```python
from build123d import *

# Parameters (mm, degrees)
BOSS_EXTRUDE1_DEPTH = 5
CUT_EXTRUDE1_DEPTH  = 2
SKETCH3_R           = 10
CUT_EXTRUDE4_DEPTH  = 73.034713854
BOSS_EXTRUDE2_START = 2
SKETCH5_R           = 15
SKETCH5_R_2         = 10
BOSS_EXTRUDE2_DEPTH = 2


with BuildPart() as part:
    # Sketch1 → Boss-Extrude1 (new, symmetric)
    with BuildSketch(Plane(origin=(0, 0, 0), x_dir=(1, 0, 0), z_dir=(0, 1, 0))):
        with BuildLine():
            Line((-28.618176043, 9), (-14.309088021, 54.5))
            ThreePointArc((-14.309088021, 54.5), (0, 65), (14.309088021, 54.5))
            Line((14.309088021, 54.5), (28.618176043, 9))
            ThreePointArc((28.618176043, 9), (0, -30), (-28.618176043, 9))
        make_face()
    extrude(amount=BOSS_EXTRUDE1_DEPTH, both=True)

    # Sketch2 → Cut-Extrude1 (cut)
    with BuildSketch(Plane(origin=(0, 5, 0), x_dir=(1, 0, 0), z_dir=(0, 1, 0))):
        with BuildLine():
            Line((-9.539392014, 53), (-23.848480035, 7.5))
            ThreePointArc((-23.848480035, 7.5), (0, -25), (23.848480035, 7.5))
            Line((23.848480035, 7.5), (9.539392014, 53))
            ThreePointArc((9.539392014, 53), (0, 60), (-9.539392014, 53))
        make_face()
    cut_extrude1 = extrude(amount=-CUT_EXTRUDE1_DEPTH, mode=Mode.SUBTRACT)

    # Mirror1: Cut-Extrude1 across plane
    add(cut_extrude1.mirror(Plane.ZX), mode=Mode.SUBTRACT)

    # Sketch3 → Cut-Extrude4 (cut, through all)
    with BuildSketch(Plane(origin=(0, 3, 0), x_dir=(1, 0, 0), z_dir=(0, 1, 0))):
        with Locations(Location((0, 0, 0), (0, 0, 270))):
            Circle(SKETCH3_R)
    extrude(amount=-CUT_EXTRUDE4_DEPTH, mode=Mode.SUBTRACT)

    # Sketch5 → Boss-Extrude2 (add)
    with BuildSketch(Plane(origin=(0, 3, 0), x_dir=(1, 0, 0), z_dir=(0, 1, 0)).offset(BOSS_EXTRUDE2_START)):
        with Locations(Location((0, 0, 0), (0, 0, 270))):
            Circle(SKETCH5_R)
        with Locations(Location((0, 0, 0), (0, 0, 270))):
            Circle(SKETCH5_R_2, mode=Mode.SUBTRACT)
    boss_extrude2 = extrude(amount=-BOSS_EXTRUDE2_DEPTH)

    # Mirror2: Boss-Extrude2 across plane
    add(boss_extrude2.mirror(Plane.ZX))


solid = part.part
```
Geometry: final body of the model. Coordinates: model frame, mm. A direction names the side the tool comes from. Coordinates: 2 decimals unless noted, no trailing zeros. Order: outer loops, then holes, each group sorted by start corner. A loop starts at its lowest first (then second) coordinate and runs counter-clockwise, first axis right, second up.
Item 1: Draft query along Z for faces 4 (the face through (0, 0, -65)), 5 (the face through (0, -3, -18)), 6 (the face through (0.79, 0.07, 29.99)). Return one class per face: released by +Z, released by -Z, zero draft, split by the parting line, or undercut.
Answer:
face 4: released by -Z
face 5: undercut
face 6: split by the parting line
Item 2: Section query A-A (x = 0). Output: boundary loops of the cut face in (y, z), then the cut area to 3 significant figures.
Answer:
outline: (-5, -65) - (5, -65) - (5, -60) - (3, -60) - (3, -15) - (5, -15) - (5, -10) - (-5, -10) - (-5, -15) - (-3, -15) - (-3, -60) - (-5, -60) - close; (-5, 10) - (5, 10) - (5, 15) - (3, 15) - (3, 25) - (5, 25) - (5, 30) - (-5, 30) - (-5, 25) - (-3, 25) - (-3, 15) - (-5, 15) - close
area: 530 mm2
Item 3: Section query D-D (z = -48). Output: boundary loops of the cut face in (x, y), then the cut area to 3 significant figures.
Answer:
outline: (-16.35, -5) - (-11.11, -5) - (-11.11, -3) - (11.11, -3) - (11.11, -5) - (16.35, -5) - (16.35, 5) - (11.11, 5) - (11.11, 3) - (-11.11, 3) - (-11.11, 5) - (-16.35, 5) - close
area: 238 mm2
Item 4: Section query B-B (y = -0.5). Output: boundary loops of the cut face in (x, z).
Answer:
outline: (-28.62, -9) - (-14.31, -54.5) arc R15 ccw to (14.31, -54.5) - (28.62, -9) arc R30 ccw (long way) to start; hole circle Ø20 at (0, 0)
Item 5: Section query C-C (z = 0). Output: boundary loops of the cut face in (x, y).
Answer:
outline: (-30, -5) - (-25, -5) - (-25, -3) - (-15, -3) - (-15, -5) - (-10, -5) - (-10, 5) - (-15, 5) - (-15, 3) - (-25, 3) - (-25, 5) - (-30, 5) - close; (10, -5) - (15, -5) - (15, -3) - (25, -3) - (25, -5) - (30, -5) - (30, 5) - (25, 5) - (25, 3) - (15, 3) - (15, 5) - (10, 5) - close
Item 6: Material intervals for line 1 along X through (y, z) = (4.3, 0); line 2 along Z through (x, y) = (-0.5, 0.5); line 3 along Z through (x, y) = (5.5, -4.5), sorted ascending.
Answer:
line 1: x = -30 to -25, -15 to -10, 10 to 15, 25 to 30
line 2: z = -64.99 to -9.99, 9.99 to 30
line 3: z = -63.96 to -58.35, -13.96 to -8.35, 8.35 to 13.96, 24.39 to 29.49
Item 7: Access query for faces 1 (the face through (0, -4, -60)), 2 (the face through (-9.76, -0.07, -2.17)), 3 (the face through (-0.66, 4.01, 24.99)). Directions: +Z, -Z, +X, -X, +Y, -Y. A direction counts if a zero-diameter tool reaches every point of the face in a straight line with its end or side. Return the directions, or none.
Answer:
face 1: -Y
face 2: +Y, -Y
face 3: +Y
Item 8: Contact query for flat-ended pins moving along their axis: P1, Ø2, axis at x = -16.5, z = -7, coming from the +Y side; P2, Ø3, axis at x = 13.5, z = -34.5, coming from the -Y side; P3, Ø1, axis at y = 0.5, z = -14, coming from the +X side. Output: stop coordinate, or through.
Answer:
P1: stops at y = 3
P2: stops at y = -3
P3: stops at x = 27.2
